```python
from build123d import *

# Parameters (mm, degrees)
SKETCH1_R           = 4
SKETCH1_W           = 195.372583002
SKETCH1_H           = 195.372583002
BOSS_EXTRUDE1_DEPTH = 4
SKETCH2_R           = 2
CUT_EXTRUDE1_DEPTH  = 10


with BuildPart() as part:
    # Sketch1 → Boss-Extrude1 (new body)
    with BuildSketch(Plane.XY):
        with BuildLine():
            Line((-109, 125), (109, 125))
            ThreePointArc((109, 125), (120.313708499, 120.313708499), (125, 109))
            Line((125, 109), (125, -109))
            ThreePointArc((125, -109), (120.313708499, -120.313708499), (109, -125))
            Line((109, -125), (-109, -125))
            ThreePointArc((-109, -125), (-120.313708499, -120.313708499), (-125, -109))
            Line((-125, -109), (-125, 109))
            ThreePointArc((-125, 109), (-120.313708499, 120.313708499), (-109, 125))
        make_face()
        with Locations((-109, 109)):
            Circle(SKETCH1_R, mode=Mode.SUBTRACT)
        with Locations((109, 109)):
            Circle(SKETCH1_R, mode=Mode.SUBTRACT)
        with Locations((109, -109)):
            Circle(SKETCH1_R, mode=Mode.SUBTRACT)
        with Locations((-109, -109)):
            Circle(SKETCH1_R, mode=Mode.SUBTRACT)
        Rectangle(SKETCH1_W, SKETCH1_H, mode=Mode.SUBTRACT)
    extrude(amount=BOSS_EXTRUDE1_DEPTH)

    # Sketch2 → Cut-Extrude1 (cut)
    with BuildSketch(Plane.XY.offset(4)):
        with Locations((-107.686291501, 83.3)):
            Circle(SKETCH2_R)
        with Locations((-107.686291501, 50)):
            Circle(SKETCH2_R)
        with Locations((-107.686291501, 16.7)):
            Circle(SKETCH2_R)
        with Locations((-107.686291501, -16.7)):
            Circle(SKETCH2_R)
        with Locations((-107.686291501, -50)):
            Circle(SKETCH2_R)
        with Locations((-107.686291501, -83.3)):
            Circle(SKETCH2_R)
        with Locations((107.686291501, -83.3)):
            Circle(SKETCH2_R)
        with Locations((107.686291501, -50)):
            Circle(SKETCH2_R)
        with Locations((107.686291501, -16.7)):
            Circle(SKETCH2_R)
        with Locations((107.686291501, 16.7)):
            Circle(SKETCH2_R)
        with Locations((107.686291501, 50)):
            Circle(SKETCH2_R)
        with Locations((107.686291501, 83.3)):
            Circle(SKETCH2_R)
    extrude(amount=-CUT_EXTRUDE1_DEPTH, mode=Mode.SUBTRACT)


solid = part.part
```
Could you check a few things on this model? Use its own coordinates, in mm. Coordinates: 2 decimals unless noted, no trailing zeros. Order: outer loops, then holes, each group sorted by start corner. A loop starts at its lowest first (then second) coordinate and runs counter-clockwise, first axis right, second up. Notation, with made-up numbers: M 20,-23.75 L 29,-23.75 A9 ccw 29,-6.75 Z; hole C -10,30.5 d2. An arc over 180 degrees is marked long. Use a Markdown table: item, result. Add a question column.
Q1. I'm going to push flat-ended pins straight in: pin 1 (10.5 mm diameter, centred on x = 109, y = -109, fed in from -Z); pin 2 (3.5 mm diameter, centred on x = 107.69, y = -83.3, fed in from +Z). Where does each tip first touch, or does it pass through?
Q2. I want a section at B-B on y = -29. List the corners of the cut face in (x, z) for me.
Q3. I want a section at A-A on z = 1.8. Give the number of separate pieces and of enclosed holes in the cut face, then the cut area to 3 significant figures.
Q4. We'd pull the mould along Y, two halves only. Please class faces 1 (the cylindrical face through (-120.437, 120.189, 1.972)), 2 (the cylindrical face through (-109.521, 112.966, 1.972)), 3 (the cylindrical face through (108.479, 112.966, 1.972)), 4 (the flat face through (102, -9, 4)): pulls with the +Y half, pulls with the -Y half, needs draft (parallel to the pull), parting line crosses it, or undercut.
Q5. If I drill on L1, parallel to X at y = 16.5, z = 3.7; L2, parallel to Y at x = 35, z = 2.15, over which ranges is the centre line in solid material (lowest first)?
Checked values:
| question | item | result |
|---|---|---|
| 1 | pin 1 | z = 0 |
| 1 | pin 2 | through |
| 2 | outline | M -125,0 L -97.69,0 L -97.69,4 L -125,4 Z; M 97.69,0 L 125,0 L 125,4 L 97.69,4 Z |
| 3 | separate pieces | 1 |
| 3 | enclosed holes | 17 |
| 3 | area | 23,800 mm² |
| 4 | face 1 | pulls with the +Y half |
| 4 | face 2 | undercut |
| 4 | face 3 | undercut |
| 4 | face 4 | needs draft |
| 5 | L1 | -125 to -109.68, -105.7 to -97.69, 97.69 to 105.7, 109.68 to 125 |
| 5 | L2 | -125 to -97.69, 97.69 to 125 |
